from build123d import *

# Parameters (mm, degrees)
F0_R     = 75
F1_DEPTH = 80
F2_R     = 25
F3_R     = 44
F4_DEPTH = 177.9


with BuildPart() as f1:
    # F0 (on Top) → F1 (new body)
    with BuildSketch(Plane.XY):
        Circle(F0_R)
    extrude(amount=F1_DEPTH)

    # F2
    f2_edges = [f1.edges().sort_by_distance(p)[0] for p in [
        (75, 0, 40),
        (-75, 0, 0),
        (-75, 0, 80),
    ]]
    fillet(f2_edges, radius=F2_R)

    # F3 (on face) → F4 (cut)
    with BuildSketch(Plane.XY.offset(80)):
        Circle(F3_R)
    extrude(amount=-F4_DEPTH, mode=Mode.SUBTRACT)


solid = f1.part
The listing builds one solid part. Answer for the finished solid, in the listing's coordinates (mm). Round coordinates to 2 decimals unless told otherwise and drop trailing zeros. Write each loop counter-clockwise with the first axis right and the second up, starting at its lowest first coordinate (ties: lowest second). Pieces come first, ordered by that corner, then holes. Notation, with made-up numbers: (-32.5, 48.25) - (-0.5, 48.25) arc R37 cw to (-0.5, 84.25) - close; hole circle Ø4 at (-30, 80). An arc over 180 degrees is marked (long way). Use one line per item in the form item = value. Start each with the question number.
Item 1: Flat-ended cylindrical pins translate along their axes: pin 1 Ø3 at (y, z) = (50.5, 24) entering from +X; pin 2 Ø8 at (x, z) = (49, 11) entering from +Y; pin 3 Ø8 at (y, z) = (-10, 70) entering from -X. Find the tip coordinate at first contact, or state that the pin passes through.
Item 2: A cutting plane is placed at D-D (z = 5.5). Write down the section's boundary in (x, y).
Item 3: Determine the mould class of faces 1 (the cylindrical face through (-9.538, -42.954, 40.56)), 2 (the cylindrical face through (-9.764, 74.362, 39.79)), 3 (the flat face through (-0.2, -44.2, 80)) for opening direction X: +X half, -X half, draft (parallel to the pull), parting line (faces both ways), or undercut.
Item 4: Find the intervals of material crossed by line 1 (Y direction, x = 0, z = 40); line 2 (X direction, y = -10.5, z = 46.5); line 3 (X direction, y = 37, z = 4), in increasing order. Write a range as [from, to].
Item 5: A cutting plane is placed at C-C (z = 37.5). Write down the section's boundary in (x, y).
Item 6: A cutting plane is placed at A-A (y = 0). Write down the section's boundary in (x, z), plus the area to 3 significant figures.
The answers:
q1.pin_1 = 56.76
q1.pin_2 = 55.75
q1.pin_3 = -71.83
q2.outline = circle Ø131.29 at (0, 0); hole circle Ø88 at (0, 0)
q3.face_1 = undercut
q3.face_2 = parting line
q3.face_3 = draft
q4.line_1 = [-75, -44], [44, 75]
q4.line_2 = [-74.26, -42.73], [42.73, 74.26]
q4.line_3 = [-51.69, -23.81], [23.81, 51.69]
q5.outline = circle Ø150 at (0, 0); hole circle Ø88 at (0, 0)
q6.outline = (-75, 25) arc R25 ccw to (-50, 0) - (-44, 0) - (-44, 80) - (-50, 80) arc R25 ccw to (-75, 55) - close; (44, 0) - (50, 0) arc R25 ccw to (75, 25) - (75, 55) arc R25 ccw to (50, 80) - (44, 80) - close
q6.area = 4,420 mm^2
